```python
from build123d import *

# Parameters (mm, degrees)
ESQUISSE5_W                  = 4.75
ESQUISSE5_H                  = 4.75
BOSS_EXTRU_3_DEPTH           = 4
BOSS_EXTRU_4_DEPTH           = 4
ENL_V_MAT_EXTRU_1_DEPTH      = 40
ENL_V_MAT_EXTRU_1_DEPTH_BACK = 30
ESQUISSE7_R                  = 4.5


with BuildPart() as part:
    # Esquisse1 → Révolution1 (revolve)
    with BuildSketch(Plane(origin=(0, 0, 0), x_dir=(1, 0, 0), z_dir=(0, 1, 0))):
        Polygon((0, 0), (0, 4.75), (159, 4.75), (159, 0), (136.25, 0), (104.5, -9), (54.5, -9), (22.75, 0), align=None)
    revolve(axis=Axis((0, 0, -4.75), (1, 0, 0)))

    # Esquisse5 → Boss.-Extru.3 (add)
    with BuildSketch(Plane(origin=(159, 0, 0), x_dir=(0, 0, -1), z_dir=(1, 0, 0))):
        with Locations((4.75, 0)):
            Rectangle(ESQUISSE5_W, ESQUISSE5_H)
    extrude(amount=BOSS_EXTRU_3_DEPTH)

    # Esquisse6 → Boss.-Extru.4 (add)
    with BuildSketch(Plane.ZY):
        Polygon((-4.75, 2.375), (-7.125, 2.375), (-7.125, -2.375), (-2.375, -2.375), (-2.375, 2.375), align=None)
    extrude(amount=BOSS_EXTRU_4_DEPTH)

    # Esquisse7 → Enlèv. mat.-Extru.1 (cut, two sides: drawn at the far end of the back side and taken through both)
    with BuildSketch(Plane.XY.offset(-2.375).offset(-ENL_V_MAT_EXTRU_1_DEPTH_BACK)):
        with Locations(Location((79.5, 0, 0), (0, 0, 179.999999999))):
            Circle(ESQUISSE7_R)
    extrude(amount=ENL_V_MAT_EXTRU_1_DEPTH + ENL_V_MAT_EXTRU_1_DEPTH_BACK, mode=Mode.SUBTRACT)


solid = part.part
```
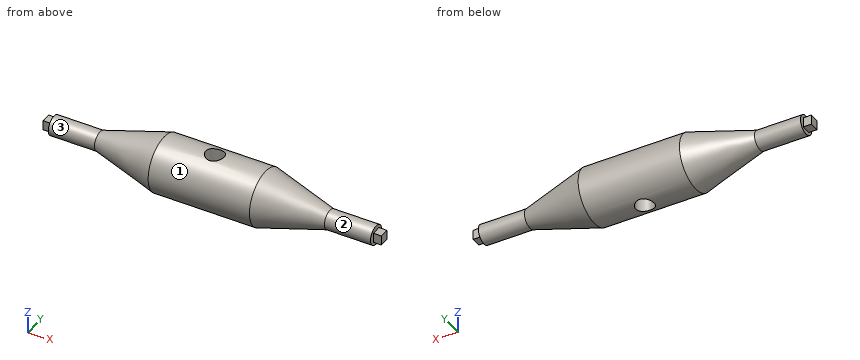
Design review of the part built by this model. Coordinates are the model's own, in mm. Face numbers are marked on the shaded views. A direction names the side the tool comes from. Coordinates: 2 decimals unless noted, no trailing zeros. Loops run counter-clockwise (first coordinate to the right, second up) from the corner with the lowest first, then second, coordinate; pieces in that order, holes last. Notation, with made-up numbers: (-28.5, 35) - (0.5, 35) arc R28 cw to (0.5, 68) - close; hole circle Ø5 at (50.5, 83). An arc over 180 degrees is marked (long way). Use CSV: the item, a comma, the result in double quotes. Start each with the question number.
1) For pin 1 Ø1.2 at (x, z) = (161.5, -6) entering from +Y (3 decimals); pin 2 Ø4.5 at (x, y) = (-1, -1) entering from +Z; pin 3 Ø1.2 at (x, y) = (161.5, 0) entering from +Z (3 decimals), all flat-tipped, find the tip position at first contact; note any pin that passes through.
2) Tool access review of the marked faces 1, 2 and 3: name each direction out of +Z, -Z, +X, -X, +Y, -Y from which nothing blocks a thin tool from reaching the whole face with its end or side.
3) Consider section A-A on z = -4.75. Write out the cut boundary in (x, y) (3 decimals).
4) Consider section B-B on y = 0. Write out the cut boundary in (x, z) (3 decimals).
5) Consider section D-D on x = 79.5. Write out the cut boundary in (y, z), then the cut area to 3 significant figures.
6) Wall thickness on L1, parallel to Y at x = 79.5, z = -4.75; L2, parallel to Y at x = 79.5, z = 3; L3, parallel to Y at x = 67, z = -4: over which ranges is each line inside the solid? List them lowest first. Write a range as from..to.
7) Consider section C-C on x = 16.5. Write out the cut boundary in (y, z), then the cut area to 3 significant figures.
Geometry says:
1,pin 1,"y = 2.375"
1,pin 2,"z = 0"
1,pin 3,"z = -2.375"
2,face 1,"+X, -X"
2,face 2,"+X"
2,face 3,"-X"
3,outline,"(-4, -2.375) - (0, -2.375) - (0, -4.75) - (22.75, -4.75) - (54.5, -13.75) - (104.5, -13.75) - (136.25, -4.75) - (159, -4.75) - (159, -2.375) - (163, -2.375) - (163, 2.375) - (159, 2.375) - (159, 4.75) - (136.25, 4.75) - (104.5, 13.75) - (54.5, 13.75) - (22.75, 4.75) - (0, 4.75) - (0, 2.375) - (-4, 2.375) - close; hole circle Ø9 at (79.5, 0)"
4,outline,"(-4, -7.125) - (0, -7.125) - (0, -9.5) - (22.75, -9.5) - (54.5, -18.5) - (75, -18.5) - (75, 9) - (54.5, 9) - (22.75, 0) - (0, 0) - (0, -2.375) - (-4, -2.375) - close; (84, -18.5) - (104.5, -18.5) - (136.25, -9.5) - (159, -9.5) - (159, -7.125) - (163, -7.125) - (163, -2.375) - (159, -2.375) - (159, 0) - (136.25, 0) - (104.5, 9) - (84, 9) - close"
5,outline,"(-4.5, -17.74) - (-4.5, 8.24) arc R13.75 ccw to start; (4.5, -17.74) arc R13.75 ccw to (4.5, 8.24) - close"
5,area,"351 mm^2"
6,L1,"-13.75..-4.5, 4.5..13.75"
6,L2,"-11.36..-4.5, 4.5..11.36"
6,L3,"-13.73..13.73"
7,outline,"circle Ø9.5 at (0, -4.75)"
7,area,"70.9 mm^2"
